Verification items for the finished model (mm, model axes). A direction names the side the tool comes from. Coordinates: 2 decimals unless noted, no trailing zeros. Write each loop counter-clockwise with the first axis right and the second up, starting at its lowest first coordinate (ties: lowest second). Pieces come first, ordered by that corner, then holes. Notation, with made-up numbers: M 87,3 L 121,3 A19 ccw 121,12 Z; hole C -12,20 d10. An arc over 180 degrees is marked long. One line per item, written item: value.
```python
from build123d import *

# Parameters (mm, degrees)
SKETCH_1_W          = 31.48
SKETCH_1_H          = 26.5
SKETCH_1_R          = 1.1
SKETCH_1_R_2        = 1.6
EXTRUDE_1_DEPTH     = 3
SKETCH_2_W          = 17.48
SKETCH_2_H          = 18.5
CUT_EXTRUDE_1_DEPTH = 21.5
FILLET_1_R          = 7
CUT_EXTRUDE_2_DEPTH = 21.5
FILLET_2_R          = 1.5


with BuildPart() as part:
    # 草图1 → 凸台-拉伸1 (new body)
    with BuildSketch(Plane(origin=(0, 0, 0), x_dir=(1, 0, 0), z_dir=(0, 1, 0))):
        with Locations((12.74, -4.25)):
            Rectangle(SKETCH_1_W, SKETCH_1_H)
        with Locations(Location((0, 7, 0), (0, 0, 270))):
            Circle(SKETCH_1_R, mode=Mode.SUBTRACT)
        with Locations(Location((7, 0, 0), (0, 0, 270))):
            Circle(SKETCH_1_R, mode=Mode.SUBTRACT)
        with Locations(Location((0, -7, 0), (0, 0, 270))):
            Circle(SKETCH_1_R, mode=Mode.SUBTRACT)
        with Locations(Location((3.48, -14.5, 0), (0, 0, 270))):
            Circle(SKETCH_1_R_2, mode=Mode.SUBTRACT)
        with Locations(Location((23.48, -14.5, 0), (0, 0, 270))):
            Circle(SKETCH_1_R_2, mode=Mode.SUBTRACT)
    extrude(amount=EXTRUDE_1_DEPTH)

    # 草图2 → 切除-拉伸1 (cut)
    with BuildSketch(Plane(origin=(0, 3, 0), x_dir=(1, 0, 0), z_dir=(0, 1, 0))):
        with Locations((19.74, -0.25)):
            Rectangle(SKETCH_2_W, SKETCH_2_H)
        with BuildLine():
            Line((-1, 4.387482194), (-1, -4.387482194))
            ThreePointArc((-1, -4.387482194), (4.5, 0), (-1, 4.387482194))
        make_face()
    extrude(amount=-CUT_EXTRUDE_1_DEPTH, mode=Mode.SUBTRACT)

    # 圆角1
    fillet_1_edges = [part.edges().sort_by_distance(p)[0] for p in [
        (11, 1.5, -9),
        (11, 1.5, 9.5),
    ]]
    fillet(fillet_1_edges, radius=FILLET_1_R)

    # 草图3 → 切除-拉伸2 (cut)
    with BuildSketch(Plane(origin=(0, 3, 0), x_dir=(1, 0, 0), z_dir=(0, 1, 0))):
        with BuildLine():
            Line((7.48, -7.5), (7.48, -15.5))
            Line((7.48, -15.5), (19.48, -15.5))
            Line((19.48, -15.5), (19.48, -12.389873609))
            ThreePointArc((19.48, -12.389873609), (13.656415306, -11.507400958), (9.339745962, -7.5))
            Line((9.339745962, -7.5), (7.48, -7.5))
        make_face()
    extrude(amount=-CUT_EXTRUDE_2_DEPTH, mode=Mode.SUBTRACT)

    # 圆角2
    # the kernel refuses this fillet: 1.5 mm, written as the material it adds along each edge
    with BuildSketch(Plane(origin=(-1, 3, -4.387482194), x_dir=(0, 0, 1), z_dir=(0, -1, 0))) as fillet_2_piece_1:
        with BuildLine():
            CenterArc((1.429442302, -1.5), FILLET_2_R, 90, 99.594068227)
            ThreePointArc((-0.049577644, -1.75), (-0.110713057, -0.872565759), (0, 0))
            Line((0, 0), (1.429442302, 0))
        make_face()
    extrude(amount=3)
    with BuildSketch(Plane(origin=(-1, 3, 4.387482194), x_dir=(0, 0, -1), z_dir=(0, -1, 0))) as fillet_2_piece_2:
        with BuildLine():
            CenterArc((1.429442302, 1.5), FILLET_2_R, 170.405931773, 99.594068227)
            ThreePointArc((-0.049577644, 1.75), (-0.110713057, 0.872565759), (0, 0))
            Line((0, 0), (1.429442302, 0))
        make_face()
    extrude(amount=3)
    with BuildSketch(Plane(origin=(19.48, 3, 12.389873609), x_dir=(-0.9973071885231932, 0, 0.07333738282733993), z_dir=(0, -1, 0))) as fillet_2_piece_3:
        with BuildLine():
            CenterArc((1.614041963, -1.495767206), FILLET_2_R, 94.30534313, 89.900355116)
            Line((0.11808118, -1.60577328), (0, 0))
            ThreePointArc((0, 0), (0.750717192, -0.02821863), (1.501434384, 0))
        make_face()
    extrude(amount=3)
    with BuildSketch(Plane(origin=(19.48, 3, 15.5), x_dir=(0, 0, -1), z_dir=(0, -1, 0)), Plane(origin=(7.48, 3, 7.5), x_dir=(0, 0, 1), z_dir=(0, -1, 0))) as fillet_2_piece_4:
        with BuildLine():
            CenterArc((FILLET_2_R, -FILLET_2_R), FILLET_2_R, 90, 90)
            Line((0, -FILLET_2_R), (0, 0))
            Line((0, 0), (FILLET_2_R, 0))
        make_face()
    extrude(amount=3)
    with BuildSketch(Plane(origin=(7.48, 3, 15.5), x_dir=(0, 0, -1), z_dir=(0, -1, 0))) as fillet_2_piece_5:
        with BuildLine():
            CenterArc((FILLET_2_R, FILLET_2_R), FILLET_2_R, 180, 90)
            Line((0, FILLET_2_R), (0, 0))
            Line((0, 0), (FILLET_2_R, 0))
        make_face()
    extrude(amount=3)
    with BuildSketch(Plane(origin=(9.339745962, 3, 7.5), x_dir=(-1, 0, 0), z_dir=(0, -1, 0))) as fillet_2_piece_6:
        with BuildLine():
            CenterArc((0.826578943, -1.5), FILLET_2_R, 90, 55.58261129)
            ThreePointArc((-0.410834055, -0.652173913), (-0.199131088, -0.330046756), (0, 0))
            Line((0, 0), (0.826578943, 0))
        make_face()
    extrude(amount=3)
    # the kernel refuses this fillet: 1.5 mm, written as the material it takes off along each edge
    with BuildSketch(Plane(origin=(28.48, 6.75, 9.5), x_dir=(-1, 0, 0), z_dir=(0, -1, 0)), Plane(origin=(-3, -3.75, 17.5), x_dir=(0, 0, -1), z_dir=(0, 1, 0)), Plane(origin=(-3, -3.75, -9), x_dir=(1, 0, 0), z_dir=(0, 1, 0))) as fillet_2_2_piece_1:
        with BuildLine():
            CenterArc((FILLET_2_R, -FILLET_2_R), FILLET_2_R, 90, 90)
            Line((0, -FILLET_2_R), (0, 0))
            Line((0, 0), (FILLET_2_R, 0))
        make_face()
    extrude(amount=10.5, mode=Mode.SUBTRACT)
    with BuildSketch(Plane(origin=(28.48, -3.75, 17.5), x_dir=(0, 0, -1), z_dir=(0, 1, 0))) as fillet_2_2_piece_2:
        with BuildLine():
            CenterArc((FILLET_2_R, FILLET_2_R), FILLET_2_R, 180, 90)
            Line((0, FILLET_2_R), (0, 0))
            Line((0, 0), (FILLET_2_R, 0))
        make_face()
    extrude(amount=10.5, mode=Mode.SUBTRACT)


solid = part.part
```
Item 1: Scan lines: line 1 (X direction, y = 1.75, z = 0); line 2 (X direction, y = 2.4, z = 15); line 3 (Z direction, x = 3, y = 1.45). Record each from-to range of solid material in increasing order.
The answers:
line 1: x = -3 to -1, 4.5 to 5.9, 8.1 to 11
line 2: x = -3 to 1.96, 5 to 7.86, 19.1 to 21.96, 25 to 28.48
line 3: z = -9 to -3.35, 3.35 to 12.97, 16.03 to 17.5
Item 2: Access from +Z, -Z, +X, -X, +Y, -Y to the whole of each face (thin tool, end or side, straight path). Record for faces 4 (the face through (1, 1, -9)), 5 (the face through (7.48, 2, 11)), 6 (the face through (22, 2, 9.5)).
The answers:
face 4: -Z, +X, -X, +Y, -Y
face 5: +Y, -Y
face 6: -Z, +X, +Y, -Y
Item 3: Cross-section at A-A, the plane x = 17.5. Enter the section's corners in (y, z).
The answers:
outline: M 0,9.48 L 3,9.48 L 3,12.49 L 0,12.49 Z; M 0,15.5 L 3,15.5 L 3,17.5 L 0,17.5 Z
Item 4: Cross-section at B-B, the plane z = -7. Enter the section's corners in (x, y).
The answers:
outline: M -3,0 L -1.1,0 L -1.1,3 L -3,3 Z; M 1.1,0 L 8.9,0 L 8.9,3 L 1.1,3 Z
Item 5: Draft check along Z on faces 1 (the face through (8.9, 1.5, -7)), 2 (the face through (-0.45, 1.52, 4.12)), 3 (the face through (9, 3, 7)). Enter one of: released by +Z, released by -Z, zero draft, split by the parting line, or undercut.
The answers:
face 1: released by -Z
face 2: undercut
face 3: zero draft
Item 6: Go/stop test with flat-tipped pins: P1, Ø1.5, axis at x = 22, y = 1.5, coming from the -Z side; P2, Ø0.9, axis at y = 2, z = 1, coming from the +X side. Record where each tip stops, or that it passes through.
The answers:
P1: stops at z = 9.5
P2: stops at x = 11
Item 7: Cross-section at C-C, the plane y = 0.65. Give the number of separate pieces and of enclosed holes in the cut face, and give its area (3 significant figures).
The answers:
separate pieces: 1
enclosed holes: 7
area: 386 mm²
Item 8: Cross-section at D-D, the plane z = 14.5. Enter the section's corners in (x, y), and give its area (3 significant figures).
The answers:
outline: M -3,0 L 1.88,0 L 1.88,3 L -3,3 Z; M 5.08,0 L 7.57,0 L 7.57,3 L 5.08,3 Z; M 19.39,0 L 21.88,0 L 21.88,3 L 19.39,3 Z; M 25.08,0 L 28.48,0 L 28.48,3 L 25.08,3 Z
area: 39.8 mm²
